```python
from build123d import *

# Parameters (mm, degrees)
CYLINDER115_R             = 6
CYLINDER115_DEPTH         = 38
CYLINDER114_R             = 11
CYLINDER114_DEPTH         = 7
FUSION033_PLACEMENT_ANGLE = 90
CYLINDER102_R             = 6
CYLINDER102_DEPTH         = 10
CYLINDER104_R             = 11
CYLINDER104_DEPTH         = 7
CYLINDER103_R             = 15
CYLINDER103_DEPTH         = 10
CUT114_PLACEMENT_ANGLE    = 90
CYLINDER112_R             = 28
CYLINDER112_DEPTH         = 30
CYLINDER113_R             = 33
CYLINDER113_DEPTH         = 30


with BuildPart() as center_cylinder043:
    # Cylinder115 → Cylinder115 (new body)
    with BuildSketch(Plane.XY.offset(-9)):
        Circle(CYLINDER115_R)
    extrude(amount=CYLINDER115_DEPTH)


with BuildPart() as fusion033:
    # Cylinder114 → Cylinder114 (new body)
    with BuildSketch(Plane.XY.offset(8)):
        Circle(CYLINDER114_R)
    extrude(amount=CYLINDER114_DEPTH)

    # Fusion033: union center-Cylinder043
    add(center_cylinder043.part)


with BuildPart() as fusion033_1:
    # Fusion033 placement: moved
    add(fusion033.part.rotate(Axis((0, 0, 0), (0, 1, 0)), FUSION033_PLACEMENT_ANGLE))


with BuildPart() as center_cylinder039:
    # Cylinder102 → Cylinder102 (new body)
    with BuildSketch(Plane.XY.offset(5)):
        Circle(CYLINDER102_R)
    extrude(amount=CYLINDER102_DEPTH)


with BuildPart() as center_cylinder041:
    # Cylinder104 → Cylinder104 (new body)
    with BuildSketch(Plane.XY.offset(8)):
        Circle(CYLINDER104_R)
    extrude(amount=CYLINDER104_DEPTH)


with BuildPart() as cut114:
    # Cylinder103 → Cylinder103 (new body)
    with BuildSketch(Plane.XY.offset(5)):
        Circle(CYLINDER103_R)
    extrude(amount=CYLINDER103_DEPTH)

    # Cut113: cut center-Cylinder041
    add(center_cylinder041.part, mode=Mode.SUBTRACT)

    # Cut114: cut center-Cylinder039
    add(center_cylinder039.part, mode=Mode.SUBTRACT)


with BuildPart() as cut114_1:
    # Cut114 placement: moved
    add(cut114.part.rotate(Axis((0, 0, 0), (0, 1, 0)), CUT114_PLACEMENT_ANGLE))


with BuildPart() as cylinder112:
    # Cylinder112 → Cylinder112 (new body)
    with BuildSketch(Plane(origin=(-23, 0, -2), x_dir=(1, 0, 0), z_dir=(0, 0, 1))):
        Circle(CYLINDER112_R)
    extrude(amount=CYLINDER112_DEPTH)


with BuildPart() as cut120:
    # Cylinder113 → Cylinder113 (new body)
    with BuildSketch(Plane(origin=(-23, 0, -2), x_dir=(1, 0, 0), z_dir=(0, 0, 1))):
        Circle(CYLINDER113_R)
    extrude(amount=CYLINDER113_DEPTH)

    # Cut119: cut Cylinder112
    add(cylinder112.part, mode=Mode.SUBTRACT)

    # Fusion034: union Cut114
    add(cut114_1.part)

    # Cut120: cut Fusion033
    add(fusion033_1.part, mode=Mode.SUBTRACT)


solid = cut120.part
```
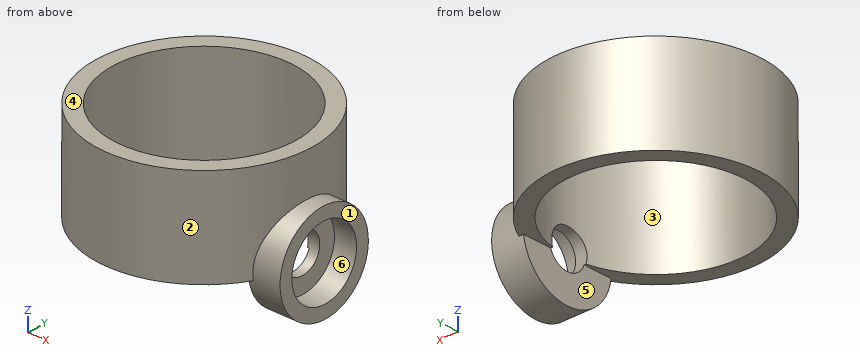
For this review, take the finished solid that the model builds, in its own axes (mm). Face numbers are marked on the shaded views. A direction names the side the tool comes from. Coordinates: 2 decimals unless noted, no trailing zeros. Loops run counter-clockwise (first coordinate to the right, second up) from the corner with the lowest first, then second, coordinate; pieces in that order, holes last. Notation, with made-up numbers: (25, 20.25) - (48, 20.25) arc R28 ccw to (48, 51.25) - close; hole circle Ø10 at (75.5, 58). An arc over 180 degrees is marked (long way). Use one line per item in the form item = value. Start each with the question number.
1) Take a section at C-C (y = 14). State the section outline as (x, z) points.
2) Take a section at A-A (x = -23). State the section outline as (y, z) points.
3) Take a section at B-B (y = 0). State the section outline as (x, z) points, plus the area to 3 significant figures.
4) Draft analysis for pull direction Y (two halves, no side actions). For the marked faces 1, 2 and 3, state which applies: released by +Y, released by -Y, zero draft, split by the parting line, or undercut.
5) For pin 1 (6 mm diameter, centred on y = -20.5, z = -2.5, fed in from -X); pin 2 (1.5 mm diameter, centred on y = -15.5, z = 6.5, fed in from -X); pin 3 (1.5 mm diameter, centred on x = -13.5, z = -3, fed in from -Y); pin 4 (6.5 mm diameter, centred on y = 7, z = -7, fed in from -X), all flat-tipped, find the tip position at first contact; note any pin that passes through.
6) To check wall thickness, follow probe 1 along X at (y, z) = (0, 21); probe 2 along Y at (x, z) = (-23, 15.5); probe 3 along Z at (x, y) = (5.35, 0). State the ranges of each line that lie inside material, in increasing order. Write a range as from..to.
7) Take a section at D-D (z = 21). State the section outline as (x, y) points.
8) For the marked faces 4, 5 and 6, list the 3-axis set-ups (+Z, -Z, +X, -X, +Y, -Y) from which the entire face can be reached by the end or side of a thin tool; tool diameter is ignored.
From the geometry:
q1.outline = (-52.88, -2) - (-47.25, -2) - (-47.25, 28) - (-52.88, 28) - close; (1.25, -2) - (5, -2) - (5, -5.39) - (15, -5.39) - (15, 5.39) - (6.88, 5.39) - (6.88, 28) - (1.25, 28) - close
q2.outline = (-33, -2) - (-28, -2) - (-28, 28) - (-33, 28) - close; (28, -2) - (33, -2) - (33, 28) - (28, 28) - close
q3.outline = (-56, -2) - (-51, -2) - (-51, 28) - (-56, 28) - close; (5, -15) - (15, -15) - (15, -11) - (8, -11) - (8, -6) - (5, -6) - close; (5, 6) - (8, 6) - (8, 11) - (15, 11) - (15, 15) - (10, 15) - (10, 28) - (5, 28) - close
q3.area = 325 mm2
q4.face_1 = zero draft
q4.face_2 = split by the parting line
q4.face_3 = undercut
q5.pin_1 = -50.95
q5.pin_2 = -52.52
q5.pin_3 = through
q5.pin_4 = 5
q6.probe_1 = -56..-51, 5..10
q6.probe_2 = -33..-28, 28..33
q6.probe_3 = -15..-6, 6..28
q7.outline = circle Ø66 at (-23, 0); hole circle Ø56 at (-23, 0)
q8.face_4 = +Z, +X, -X, +Y, -Y
q8.face_5 = -Z, -X, +Y, -Y
q8.face_6 = +X
